The model under review builds one solid part; all positions refer to its coordinate system, in mm. Face numbers are marked on the shaded views. A direction names the side the tool comes from. Coordinates: 2 decimals unless noted, no trailing zeros. Loops run counter-clockwise (first coordinate to the right, second up) from the corner with the lowest first, then second, coordinate; pieces in that order, holes last. Notation, with made-up numbers: M 76.25,32 L 89.25,32 A22 cw 89.25,65 Z; hole C -23.5,-1.5 d9. An arc over 180 degrees is marked long. Return JSON: item names as keys, results as strings.
```python
from build123d import *

# Parameters (mm, degrees)
SKETCH1_W            = 558.8
SKETCH1_H            = 152.4
SKETCH1_W_2          = 552.45
SKETCH1_H_2          = 146.05
BOSS_EXTRUDE2_DEPTH  = 101.6
BOSS_EXTRUDE3_REACH  = 151.225
SKETCH5_W            = 552.45
SKETCH5_H            = 146.05
BOSS_EXTRUDE15_DEPTH = 12.7
SKETCH8_R            = 19.05
CUT_EXTRUDE1_DEPTH   = 102.6
SKETCH9_W            = 32.035224234
SKETCH9_H            = 127
CUT_EXTRUDE2_DEPTH   = 546.1


with BuildPart() as part:
    # Sketch1 → Boss-Extrude2 (new body)
    with BuildSketch(Plane.XY):
        with Locations((279.4, 76.2)):
            Rectangle(SKETCH1_W, SKETCH1_H)
        with Locations((279.4, 76.2)):
            Rectangle(SKETCH1_W_2, SKETCH1_H_2, mode=Mode.SUBTRACT)
    extrude(amount=BOSS_EXTRUDE2_DEPTH)

    # Sketch2 → Boss-Extrude3 (add, up to next)
    with BuildSketch(Plane(origin=(0, 3.175, 0), x_dir=(1, 0, 0), z_dir=(0, 1, 0)), mode=Mode.PRIVATE) as boss_extrude3_sk1:
        Polygon((3.175, -101.6), (215.9, -12.7), (3.175, -12.7), align=None)
    boss_extrude3_tool1 = extrude(boss_extrude3_sk1.sketch, amount=BOSS_EXTRUDE3_REACH, mode=Mode.PRIVATE) - part.part
    add(boss_extrude3_tool1.solids().sort_by_distance((74.083333, 3.175, 42.333333))[0])
    # Sketch2 → Boss-Extrude3 (add, up to next)
    with BuildSketch(Plane(origin=(0, 3.175, 0), x_dir=(1, 0, 0), z_dir=(0, 1, 0)), mode=Mode.PRIVATE) as boss_extrude3_sk2:
        Polygon((342.9, -12.7), (555.625, -101.6), (555.625, -12.7), align=None)
    boss_extrude3_tool2 = extrude(boss_extrude3_sk2.sketch, amount=BOSS_EXTRUDE3_REACH, mode=Mode.PRIVATE) - part.part
    add(boss_extrude3_tool2.solids().sort_by_distance((484.716667, 3.175, 42.333333))[0])

    # Sketch5 → Boss-Extrude15 (add)
    with BuildSketch(Plane(origin=(0, 0, 12.7), x_dir=(-1, 0, 0), z_dir=(0, 0, -1))):
        with Locations((-279.4, 76.2)):
            Rectangle(SKETCH5_W, SKETCH5_H)
    extrude(amount=BOSS_EXTRUDE15_DEPTH)

    # Sketch8 → Cut-Extrude1 (cut, through all)
    with BuildSketch(Plane(origin=(0, 0, 0), x_dir=(-1, 0, 0), z_dir=(0, 0, -1))):
        with Locations((-279.4, 25.4)):
            Circle(SKETCH8_R)
    extrude(amount=-CUT_EXTRUDE1_DEPTH, mode=Mode.SUBTRACT)

    # Sketch9 → Cut-Extrude2 (cut)
    with BuildSketch(Plane(origin=(558.8, 0, 0), x_dir=(0, 0, -1), z_dir=(1, 0, 0))):
        with Locations((-72.882387883, 66.675)):
            Rectangle(SKETCH9_W, SKETCH9_H)
    extrude(amount=-CUT_EXTRUDE2_DEPTH, mode=Mode.SUBTRACT)


solid = part.part
```
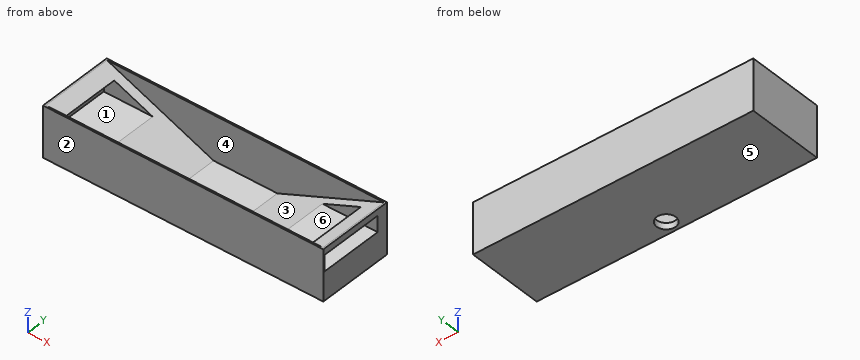
1. Add section D-D on y = 135. Give the boundary of the cut face in (x, z) (3 decimals).
Check values:
{"outline": "M 0,0 L 558.8,0 L 558.8,101.6 L 555.625,101.6 L 342.9,12.7 L 215.9,12.7 L 3.175,101.6 L 0,101.6 Z"}
2. Add section A-A on y = 25.4. Give the boundary of the cut face in (x, z) (3 decimals), plus the area to 3 significant figures.
Check values:
{"outline": "M 0,0 L 260.35,0 L 260.35,12.7 L 215.9,12.7 L 110.22,56.865 L 12.7,56.865 L 12.7,88.9 L 33.564,88.9 L 3.175,101.6 L 0,101.6 Z; M 298.45,0 L 558.8,0 L 558.8,56.865 L 448.58,56.865 L 342.9,12.7 L 298.45,12.7 Z; M 525.236,88.9 L 558.8,88.9 L 558.8,101.6 L 555.625,101.6 Z", "area": "21,900 mm²"}
3. Machinability: for the marked faces 1, 2 and 3, which of the approach directions +Z, -Z, +X, -X, +Y, -Y give a long, thin tool a straight path to every point of the face, cutting with its end or side? Answer none if there is none.
Check values:
{"face 1": "+X", "face 2": "+Z, -Z, +X, -X, -Y", "face 3": "+Z"}
4. Add section B-B on y = 88.5. Give the boundary of the cut face in (x, z) (3 decimals), plus the area to 3 significant figures.
Check values:
{"outline": "M 0,0 L 558.8,0 L 558.8,56.865 L 448.58,56.865 L 342.9,12.7 L 215.9,12.7 L 110.22,56.865 L 12.7,56.865 L 12.7,88.9 L 33.564,88.9 L 3.175,101.6 L 0,101.6 Z; M 525.236,88.9 L 558.8,88.9 L 558.8,101.6 L 555.625,101.6 Z", "area": "22,400 mm²"}
5. To check wall thickness, follow line 1 (Y direction, x = 311.5, z = 51) (3 decimals); line 2 (Y direction, x = 279.4, z = 5); line 3 (X direction, y = 25, z = 5). State the ranges of each line that lie inside material, in increasing order.
Check values:
{"line 1": "0 to 3.175, 149.225 to 152.4", "line 2": "0 to 6.35, 44.45 to 152.4", "line 3": "0 to 260.35, 298.45 to 558.8"}
6. Add section C-C on x = 279.4. Give the boundary of the cut face in (y, z) (3 decimals), plus the area to 3 significant figures.
Check values:
{"outline": "M 0,0 L 6.35,0 L 6.35,12.7 L 3.175,12.7 L 3.175,101.6 L 0,101.6 Z; M 44.45,0 L 152.4,0 L 152.4,101.6 L 149.225,101.6 L 149.225,12.7 L 44.45,12.7 Z", "area": "2,020 mm²"}
7. Insertion check: pin 1 Ø4 at (x, y) = (199, 56) entering from +Z; pin 2 Ø9.5 at (y, z) = (75, 75) entering from +X. Each pin has a flat end and moves straight along its axis. Give the tip position at first contact, or say it passes through.
Check values:
{"pin 1": "z = 20.6", "pin 2": "x = 12.7"}
8. The part is to be moulded in two halves that separate along Z. For the marked faces 4, 5 and 6, say which applies: released by +Z, released by -Z, zero draft, split by the parting line, or undercut.
Check values:
{"face 4": "zero draft", "face 5": "released by -Z", "face 6": "undercut"}
